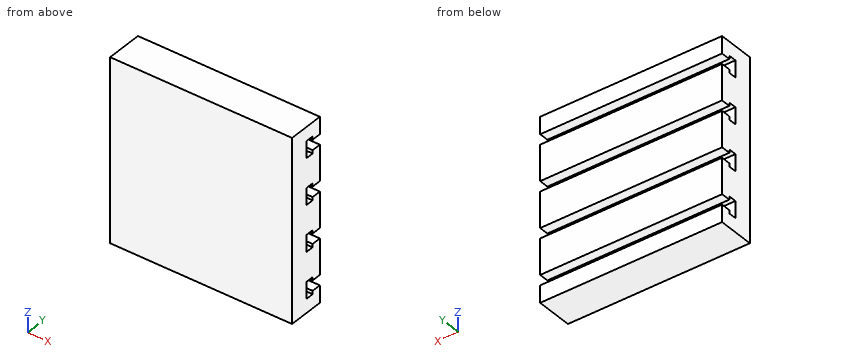
from build123d import *

# Parameters (mm, degrees)
SALIENTE_EXTRUIR1_DEPTH      = 125
SALIENTE_EXTRUIR1_DEPTH_BACK = 125
CROQUIS1_W                   = 250
CROQUIS1_H                   = 50
CORTAR_EXTRUIR1_DEPTH        = 284.94541729


with BuildPart() as part:
    # Croquis1 → Saliente-Extruir1 (new, two sides: drawn at the far end of the back side and taken through both)
    with BuildSketch(Plane(origin=(0, 0, 0), x_dir=(0, 0, -1), z_dir=(1, 0, 0)).offset(-SALIENTE_EXTRUIR1_DEPTH_BACK)):
        with Locations((0, -25)):
            Rectangle(CROQUIS1_W, CROQUIS1_H)
    extrude(amount=SALIENTE_EXTRUIR1_DEPTH + SALIENTE_EXTRUIR1_DEPTH_BACK)

    # Croquis2 → Cortar-Extruir1 (cut, through all)
    with BuildSketch(Plane(origin=(125, 0, 0), x_dir=(0, 0, -1), z_dir=(1, 0, 0))):
        Polygon((-101.5, 0), (-101.5, -13), (-106, -13), (-106, -24), (-83, -24), (-83, -13), (-87.5, -13), (-87.5, 0), align=None)
        Polygon((-24.5, 0), (-38.5, 0), (-38.5, -13), (-43, -13), (-43, -24), (-20, -24), (-20, -13), (-24.5, -13), align=None)
        Polygon((38.5, 0), (24.5, 0), (24.5, -13), (20, -13), (20, -24), (43, -24), (43, -13), (38.5, -13), align=None)
        Polygon((101.5, 0), (87.5, 0), (87.5, -13), (83, -13), (83, -24), (106, -24), (106, -13), (101.5, -13), align=None)
    extrude(amount=-CORTAR_EXTRUIR1_DEPTH, mode=Mode.SUBTRACT)


solid = part.part
Can you work these out from the model? Positions are in its coordinate system, mm. Give positions to 0.01 mm unless a question says otherwise; leave off trailing zeros. Order: outer loops, then holes, each group sorted by start corner. A loop starts at its lowest first (then second) coordinate and runs counter-clockwise, first axis right, second up. Notation, with made-up numbers: (55.5, 15.5) - (114.5, 15.5) arc R15 cw to (114.5, 25.5) - close; hole circle Ø4 at (2.5, 71). An arc over 180 degrees is marked (long way). Write each question's results on one line, items separated by ' | '.
1) I'm going to push flat-ended pins straight in: pin 1 Ø4 at (y, z) = (-16.5, 89) entering from -X; pin 2 Ø18.5 at (x, z) = (-5, -33) entering from +Y. Where does each tip first touch, or does it pass through?
Final values:
pin 1: passes through | pin 2: stops at y = 0
2) Suppose I cut it at B-B, the plane z = 34. Write out the boundary of the cut face in (x, y).
Final values:
outline: (-125, -50) - (125, -50) - (125, -24) - (-125, -24) - close
3) Suppose I cut it at A-A, the plane y = -5. Write out the boundary of the cut face in (x, z).
Final values:
outline: (-125, -125) - (125, -125) - (125, -101.5) - (-125, -101.5) - close; (-125, -87.5) - (125, -87.5) - (125, -38.5) - (-125, -38.5) - close; (-125, -24.5) - (125, -24.5) - (125, 24.5) - (-125, 24.5) - close; (-125, 38.5) - (125, 38.5) - (125, 87.5) - (-125, 87.5) - close; (-125, 101.5) - (125, 101.5) - (125, 125) - (-125, 125) - close
4) Please list where these lines run through material, in increasing order: line 1 along Z through (x, y) = (-10.5, -3); line 2 along Z through (x, y) = (-25, -21); line 3 along Y through (x, z) = (-52, -103). Write a range as [from, to].
Final values:
line 1: z = [-125, -101.5], [-87.5, -38.5], [-24.5, 24.5], [38.5, 87.5], [101.5, 125] | line 2: z = [-125, -106], [-83, -43], [-20, 20], [43, 83], [106, 125] | line 3: y = [-50, -24], [-13, 0]
